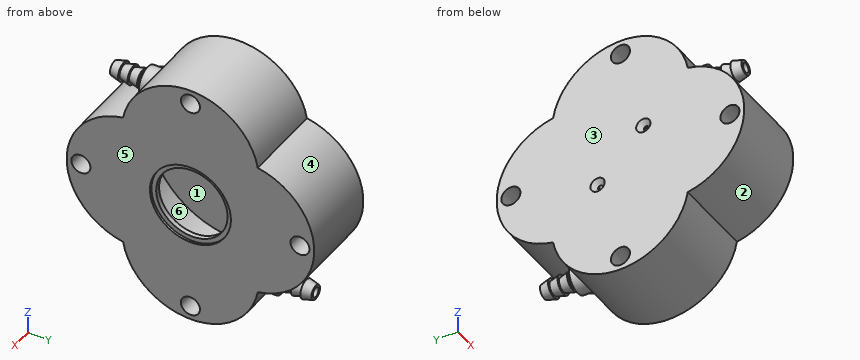
```python
from build123d import *

# Parameters (mm, degrees)
SKETCH2_R           = 2
FLANGE_DEPTH        = 8.5
SKETCH10_R          = 7.5
CUT_EXTRUDE2_DEPTH  = 10
SKETCH3_R           = 8.5
O_RING_SEAT_DEPTH   = 0.5
SKETCH8_R           = 18
CUT_EXTRUDE1_DEPTH  = 7
SKETCH5_R           = 1
OUTLET_DEPTH        = 38.739236876
BOSS_EXTRUDE2_REACH = 50.576
SKETCH6_R           = 3
SKETCH6_R_2         = 1
INLET_COUNT         = 2
SKETCH11_W          = 10.606601718
SKETCH11_H          = 10.606601718
CUT_EXTRUDE3_DEPTH  = 0.5
SKETCH12_R          = 0.5
CUT_EXTRUDE4_DEPTH  = 41.099875416
CHAMFER1_SIZE       = 1


with BuildPart() as part:
    # Sketch2 → Flange (new, symmetric)
    with BuildSketch(Plane(origin=(0, 0, 0), x_dir=(0, 0, -1), z_dir=(1, 0, 0))):
        with BuildLine():
            ThreePointArc((-14.142135624, 14.142135624), (-26, 0), (-14.142135624, -14.142135624))
            ThreePointArc((-14.142135624, -14.142135624), (0, -26), (14.142135624, -14.142135624))
            ThreePointArc((14.142135624, -14.142135624), (26, 0), (14.142135624, 14.142135624))
            ThreePointArc((14.142135624, 14.142135624), (0, 26), (-14.142135624, 14.142135624))
        make_face()
        with Locations((0, 23)):
            Circle(SKETCH2_R, mode=Mode.SUBTRACT)
        with Locations((23, 0)):
            Circle(SKETCH2_R, mode=Mode.SUBTRACT)
        with Locations((0, -23)):
            Circle(SKETCH2_R, mode=Mode.SUBTRACT)
        with Locations((-23, 0)):
            Circle(SKETCH2_R, mode=Mode.SUBTRACT)
    extrude(amount=FLANGE_DEPTH, both=True)

    # Sketch10 → Cut-Extrude2 (cut)
    with BuildSketch(Plane(origin=(8.5, 0, 0), x_dir=(0, 0, -1), z_dir=(1, 0, 0))):
        Circle(SKETCH10_R)
    extrude(amount=-CUT_EXTRUDE2_DEPTH, mode=Mode.SUBTRACT)

    # Sketch3 → O-Ring Seat (cut)
    with BuildSketch(Plane(origin=(8.5, 0, 0), x_dir=(0, 0, -1), z_dir=(1, 0, 0))):
        Circle(SKETCH3_R)
    extrude(amount=-O_RING_SEAT_DEPTH, mode=Mode.SUBTRACT)

    # Sketch8 → Cut-Extrude1 (cut, symmetric)
    with BuildSketch(Plane.ZY):
        Circle(SKETCH8_R)
    extrude(amount=CUT_EXTRUDE1_DEPTH, both=True, mode=Mode.SUBTRACT)

    # Sketch5 → Outlet (cut, through all)
    with BuildSketch(Plane(origin=(0, 0, 0), x_dir=(1, 0, 0), z_dir=(0, 1, 0))):
        with Locations(Location((0, 17, 0), (0, 0, 90))):
            Circle(SKETCH5_R)
    outlet = extrude(amount=OUTLET_DEPTH, mode=Mode.SUBTRACT)

    # Sketch6 → Boss-Extrude2 (add, up to next)
    with BuildSketch(Plane(origin=(0, 14.142135624, 0), x_dir=(1, 0, 0), z_dir=(0, 1, 0)), mode=Mode.PRIVATE) as boss_extrude2_sk1:
        with Locations((0, 17)):
            Circle(SKETCH6_R)
        with Locations(Location((0, 17, 0), (0, 0, 90))):
            Circle(SKETCH6_R_2, mode=Mode.SUBTRACT)
    boss_extrude2_tool1 = extrude(boss_extrude2_sk1.sketch, amount=-BOSS_EXTRUDE2_REACH, mode=Mode.PRIVATE) - part.part
    boss_extrude2 = boss_extrude2_tool1.solids().sort_by_distance((-2.915147, 14.142136, -17))[0]
    add(boss_extrude2)

    # Sketch9 → Revolve1 (revolve)
    with BuildSketch(Plane(origin=(0, 0, 0), x_dir=(0, 0, -1), z_dir=(1, 0, 0)), mode=Mode.PRIVATE) as revolve1_sk:
        Polygon((18, 14.142135624), (18, 21.142135624), (18.5, 21.142135624), (19, 19.142135624), (18.5, 19.142135624), (19, 17.142135624), (18.5, 17.142135624), (19, 15.142135624), (18.5, 15.142135624), (18.5, 14.142135624), align=None)
    revolve1 = revolve(revolve1_sk.sketch.rotate(Axis((0, 14.142135624, -17), (0, -1, 0)), 180), axis=Axis((0, 14.142135624, -17), (0, -1, 0)))

    # Inlet: Outlet, Boss-Extrude2, Revolve1 ×2 about axis
    inlet_axis = Axis((8, 0, 0), (1, 0, 0))
    add([outlet.rotate(inlet_axis, i * 360 / INLET_COUNT) for i in range(1, INLET_COUNT)], mode=Mode.SUBTRACT)
    add([boss_extrude2.rotate(inlet_axis, i * 360 / INLET_COUNT) for i in range(1, INLET_COUNT)])
    add([revolve1.rotate(inlet_axis, i * 360 / INLET_COUNT) for i in range(1, INLET_COUNT)])

    # Sketch11 → Cut-Extrude3 (cut)
    with BuildSketch(Plane(origin=(-7, 0, 0), x_dir=(0, 0, -1), z_dir=(1, 0, 0))):
        Rectangle(SKETCH11_W, SKETCH11_H)
    extrude(amount=-CUT_EXTRUDE3_DEPTH, mode=Mode.SUBTRACT)

    # Sketch12 → Cut-Extrude4 (cut, through all)
    with BuildSketch(Plane(origin=(-7.5, 0, 0), x_dir=(0, 0, -1), z_dir=(1, 0, 0))):
        with Locations((4.803300859, 4.803300859)):
            Circle(SKETCH12_R)
        with Locations((-4.803300859, -4.803300859)):
            Circle(SKETCH12_R)
    extrude(amount=-CUT_EXTRUDE4_DEPTH, mode=Mode.SUBTRACT)

    # Chamfer1
    chamfer1_edges = [part.edges().sort_by_distance(p)[0] for p in [
        (-8.5, 4.803300859, -4.303300859),
        (-8.5, -4.803300859, 5.303300859),
    ]]
    chamfer(chamfer1_edges, length=CHAMFER1_SIZE - 0.0001)  # a hair under: the kernel refuses the full size


solid = part.part
```
Geometry check sheet. Reference: the model listing, model coordinates, mm. Face numbers are marked on the shaded views. A direction names the side the tool comes from. Coordinates: 2 decimals unless noted, no trailing zeros. Write each loop counter-clockwise with the first axis right and the second up, starting at its lowest first coordinate (ties: lowest second). Pieces come first, ordered by that corner, then holes. Notation, with made-up numbers: M 18,73.25 L 39,73.25 A26 cw 39,87.25 Z; hole C -14.75,5 d11. An arc over 180 degrees is marked long. Use one line per item in the form item = value. Start each with the question number.
1) Thickness scan on probe 1 along X at (y, z) = (15.5, -8.5); probe 2 along Z at (x, y) = (-0.25, -9); probe 3 along Y at (x, z) = (7.75, 0.5). Record the ranges inside material, lowest first. Write a range as from..to.
2) Section check D-D on z = 0. Enter the section's corners in (x, y), and give its area (3 significant figures).
3) Section check A-A on y = -20. Enter the section's corners in (x, z).
4) Go/stop test with flat-tipped pins: pin 1 Ø2 at (y, z) = (0.5, -4) entering from +X; pin 2 Ø3.5 at (x, z) = (-0.5, 17) entering from -Y; pin 3 Ø1.8 at (x, z) = (0, 17) entering from +Y. Record where each tip stops, or that it passes through.
5) Set-up check for the marked faces 1 and 2: record each of +Z, -Z, +X, -X, +Y, -Y from which the full face is reachable in a straight line by a thin tool's end or side.
6) Section check C-C on x = -6.25. Enter the section's corners in (y, z).
7) Section check B-B on z = 23. Enter the section's corners in (x, y).
8) Release check for a two-part mould opening along X. For the marked faces 3, 4, 5 and 6 record: pulls with the +X half, pulls with the -X half, needs draft (parallel to the pull), parting line crosses it, or undercut.
Responses:
q1.probe_1 = -8.5..-7, 7..8.5
q1.probe_2 = -22.83..-15.59, 15.59..16.03, 17.97..22.83
q1.probe_3 = -25.99..-24.94, -21.06..-7.48, 7.48..21.06, 24.94..25.99
q2.outline = M -8.5,-26 L 8.5,-26 L 8.5,-25 L -8.5,-25 Z; M -8.5,-21 L 8.5,-21 L 8.5,-8.5 L 8,-8.5 L 8,-7.5 L 7,-7.5 L 7,-18 L -7,-18 L -7,-5.3 L -7.5,-5.3 L -7.5,5.3 L -7,5.3 L -7,18 L 7,18 L 7,7.5 L 8,7.5 L 8,8.5 L 8.5,8.5 L 8.5,21 L -8.5,21 Z; M -8.5,25 L 8.5,25 L 8.5,26 L -8.5,26 Z
q2.area = 215 mm2
q3.outline = M -8.5,-11.68 L 8.5,-11.68 L 8.5,11.68 L -8.5,11.68 Z; C 0,17 d3.57; hole C 0,17 d2
q4.pin_1 = -7.5
q4.pin_2 = -21.14
q4.pin_3 = 13.65
q5.face_1 = none
q5.face_2 = +X, -X, -Y
q6.outline = M -14.14,-14.14 A14.36 ccw 14.14,-14.14 A14.36 ccw 14.14,14.14 A14.36 ccw -14.14,14.14 A14.36 ccw Z; hole C -23,0 d4; hole C 0,0 d36; hole C 0,-23 d4; hole C 0,23 d4; hole C 23,0 d4
q7.outline = M -8.5,-8.78 L 8.5,-8.78 L 8.5,-2 L -8.5,-2 Z; M -8.5,2 L 8.5,2 L 8.5,8.78 L -8.5,8.78 Z
q8.face_3 = pulls with the -X half
q8.face_4 = needs draft
q8.face_5 = pulls with the +X half
q8.face_6 = undercut
